Here's how the part is built. I have some questions about the finished solid (model axes, mm). A direction names the side the tool comes from. Round coordinates to 2 decimals unless told otherwise and drop trailing zeros. Write each loop counter-clockwise with the first axis right and the second up, starting at its lowest first coordinate (ties: lowest second). Pieces come first, ordered by that corner, then holes. Notation, with made-up numbers: (64, 65.5) - (118, 65.5) arc R30 ccw to (118, 101.5) - close; hole circle Ø9 at (81, 86). An arc over 180 degrees is marked (long way). Write item = value, one per line. Start each with the question number.
Item 1: Thinking about a two-plate mould opening in X: for faces 1 (the face through (-3, 0, -10)), 2 (the face through (0.596, -2.685, -5.07)), 3 (the face through (-2.343, 17.847, 0.74)), which applies, pulls with the +X half, pulls with the -X half, needs draft (parallel to the pull), parting line crosses it, or undercut?
Item 2: For P1, Ø1, axis at x = 3, z = -4.5, coming from the -Y side; P2, Ø10, axis at x = 9.5, y = -11, coming from the -Z side; P3, Ø2, axis at y = 2.5, z = -4, coming from the -X side, each with a flat end and sliding along its axis, tell me the tip position at first contact or that it passes through.
Item 3: If I drill on line 1 along Z through (x, y) = (7.5, 10); line 2 along Y through (x, z) = (-2, -5.25); line 3 along Y through (x, z) = (0, -6.5), over which ranges is the centre line in solid material (lowest first)? Write a range as [from, to].
Item 4: If we section it at B-B (y = -12.5): Please give me the cut outline in (x, z), and give its area (3 significant figures).
Item 5: Which directions (+Z, -Z, +X, -X, +Y, -Y) give clear straight access to the entire face, cutting with the end or side of a thin tool? Please do faces 4 (the face through (0, 0, 0)), 5 (the face through (0, 0, 1.5)).
Item 6: If we section it at A-A (x = -14): Please give me the cut outline in (y, z), and give its area (3 significant figures).
```python
from build123d import *

# Parameters (mm, degrees)
SKETCH1_R           = 18
SKETCH1_R_2         = 7.5
BOSS_EXTRUDE1_DEPTH = 1.5
SKETCH2_3_R         = 2.75
CUT_EXTRUDE1_DEPTH  = 10


with BuildPart() as part:
    # Sketch1 → Boss-Extrude1 (new body)
    # profile 1 of 2: a face of its own
    with BuildSketch(Plane.XY):
        Circle(SKETCH1_R)
        Circle(SKETCH1_R_2, mode=Mode.SUBTRACT)
    # profile 2 of 2: a face of its own
    with BuildSketch(Plane.XY):
        Circle(SKETCH1_R_2)
    extrude(amount=BOSS_EXTRUDE1_DEPTH)

    # Loft1: read off the stored shape, not the designer's step
    # Loft1: loft between two sections, ruled curve by curve
    loft1_from = [
        Edge.make_bspline([(7.325491543, -1.608469353, 0), (4.108552836, -16.259452438, 0), (-10.542430249, -13.042513732, 0), (-7.325491543, 1.608469353, 0), (-4.108552836, 16.259452438, 0), (10.542430249, 13.042513732, 0), (7.325491543, -1.608469353, 0)], [0, 0, 0, 0, 0.5, 0.5, 0.5, 1, 1, 1, 1], 3, [1, 0.333333333, 0.333333333, 1, 0.333333333, 0.333333333, 1]),
    ]
    loft1_to = [
        Edge.make_bspline([(2.605092701, -1.943191195, -10), (-1.281289689, -7.153376597, -10), (-6.491475091, -3.266994207, -10), (-2.605092701, 1.943191195, -10), (1.281289689, 7.153376597, -10), (6.491475091, 3.266994207, -10), (2.605092701, -1.943191195, -10)], [0, 0, 0, 0, 0.5, 0.5, 0.5, 1, 1, 1, 1], 3, [1, 0.333333333, 0.333333333, 1, 0.333333333, 0.333333333, 1]),
    ]
    loft1 = Solid(Shell([*[Face.make_surface_from_curves(loft1_from[k], loft1_to[k]) for k in range(1)], Face(Wire(loft1_from)), Face(Wire(loft1_to))]))
    add(loft1)

    # Sketch2<3> → Cut-Extrude1 (cut)
    with BuildSketch(Plane(origin=(0, 0, -10), x_dir=(-1, 0, 0), z_dir=(0, 0, -1))):
        Circle(SKETCH2_3_R)
    extrude(amount=-CUT_EXTRUDE1_DEPTH, mode=Mode.SUBTRACT)


solid = part.part
```
Reply:
q1.face_1 = needs draft
q1.face_2 = undercut
q1.face_3 = parting line crosses it
q2.P1 = -4.99
q2.P2 = 0
q2.P3 = -5.76
q3.line_1 = [0, 1.5]
q3.line_2 = [-4.76, -1.89], [1.89, 4.76]
q3.line_3 = [-4.63, -2.75], [2.75, 4.63]
q4.outline = (-12.95, 0) - (12.95, 0) - (12.95, 1.5) - (-12.95, 1.5) - close
q4.area = 38.9 mm2
q5.face_4 = -Z
q5.face_5 = +Z, +X, -X, +Y, -Y
q6.outline = (-11.31, 0) - (11.31, 0) - (11.31, 1.5) - (-11.31, 1.5) - close
q6.area = 33.9 mm2
